```python
from build123d import *

# Parameters (mm, degrees)
SKETCH_1_W                   = 100
SKETCH_1_H                   = 50
EXTRUDE_1_DEPTH              = 10
SKETCH_2_W                   = 40
SKETCH_2_H                   = 50
EXTRUDE_2_DEPTH              = 10
FILLET_1_R                   = 10
HOLE_WIZARD_M6_1_D           = 5
HOLE_WIZARD_M6_1_CSINK_D     = 6.05
HOLE_WIZARD_M6_1_CSINK_ANGLE = 90


with BuildPart() as part:
    # 草图1 → 凸台-拉伸1 (new body)
    with BuildSketch(Plane.XY):
        Rectangle(SKETCH_1_W, SKETCH_1_H)
    extrude(amount=EXTRUDE_1_DEPTH)

    # 草图2 → 凸台-拉伸2 (add)
    with BuildSketch(Plane.XY.offset(10)):
        Rectangle(SKETCH_2_W, SKETCH_2_H)
    extrude(amount=EXTRUDE_2_DEPTH)

    # 圆角1
    fillet_1_edges = [part.edges().sort_by_distance(p)[0] for p in [
        (50, -25, 5),
        (-50, -25, 5),
        (-50, 25, 5),
        (50, 25, 5),
    ]]
    fillet(fillet_1_edges, radius=FILLET_1_R)

    # M6 螺纹孔1 (through all)
    with Locations(Plane.XY.offset(10)):
        with Locations((-40, 15), (-40, -15), (40, -15), (40, 15)):
            CounterSinkHole(HOLE_WIZARD_M6_1_D / 2, HOLE_WIZARD_M6_1_CSINK_D / 2, counter_sink_angle=HOLE_WIZARD_M6_1_CSINK_ANGLE)


solid = part.part
```
Input: part model. Units: mm. Frame: model coordinates. A direction names the side the tool comes from. Give positions to 0.01 mm unless a question says otherwise; leave off trailing zeros. Order: outer loops, then holes, each group sorted by start corner. A loop starts at its lowest first (then second) coordinate and runs counter-clockwise, first axis right, second up. Notation, with made-up numbers: M 67.5,2.25 L 101.5,2.25 A26 ccw 101.5,41.25 Z; hole C -3,89.25 d10. An arc over 180 degrees is marked long. One line per question, with ' | ' between items. Start each with the question number.
1. First-contact query: pin 1 Ø9 at (x, y) = (-33, 6.5) entering from +Z; pin 2 Ø6 at (y, z) = (-4, 15.5) entering from -X; pin 3 Ø4 at (x, y) = (40, 15) entering from +Z; pin 4 Ø3 at (y, z) = (4, 14.5) entering from +X. Flat tips, straight axial feed; report the tip coordinate or a pass-through.
2. Section query A-A (z = 6.25). Return the cut outline in (x, y), and give its area (3 significant figures).
3. Section query B-B (y = -10). Return the cut outline in (x, z).
4. Section query D-D (z = 14.25). Return the cut outline in (x, y).
5. Pull-direction query (X, two-part tool) for faces 1 (the face through (-1, 0, 0)), 2 (the face through (37.69, 14.04, 4.67)), 3 (the face through (-47.15, -21.99, 5.07)), 4 (the face through (20, 0, 15)); classes: released by +X, released by -X, zero draft, split by the parting line, or undercut.
6. Material intervals for probe 1 along Y at (x, z) = (-40, 4); probe 2 along X at (y, z) = (-15, 6.5); probe 3 along X at (y, z) = (22.5, 12), sorted ascending. Write a range as [from, to].
7. Section query C-C (x = -23). Return the cut outline in (y, z), and give its area (3 significant figures).
8. Access query for faces 5 (the face through (-50, 0, 5)), 6 (the face through (-35, 0, 10)), 7 (the face through (35, 0, 10)). Directions: +Z, -Z, +X, -X, +Y, -Y. A direction counts if a zero-diameter tool reaches every point of the face in a straight line with its end or side. Return the directions, or none.
Here are the results:
1) pin 1: z = 10 | pin 2: x = -20 | pin 3: through | pin 4: x = 20
2) outline: M -50,-15 A10 ccw -40,-25 L 40,-25 A10 ccw 50,-15 L 50,15 A10 ccw 40,25 L -40,25 A10 ccw -50,15 Z; hole C -40,-15 d5; hole C -40,15 d5; hole C 40,-15 d5; hole C 40,15 d5 | area: 4,840 mm²
3) outline: M -50,0 L 50,0 L 50,10 L 20,10 L 20,20 L -20,20 L -20,10 L -50,10 Z
4) outline: M -20,-25 L 20,-25 L 20,25 L -20,25 Z
5) face 1: zero draft | face 2: undercut | face 3: released by -X | face 4: released by +X
6) probe 1: [-25, -17.5], [-12.5, 12.5], [17.5, 25] | probe 2: [-50, -42.5], [-37.5, 37.5], [42.5, 50] | probe 3: [-20, 20]
7) outline: M -25,0 L 25,0 L 25,10 L -25,10 Z | area: 500 mm²
8) face 5: +Z, -Z, -X, +Y, -Y | face 6: +Z, -X, +Y, -Y | face 7: +Z, +X, +Y, -Y
